from build123d import *

# Parameters (mm, degrees)
SKETCH1_R               = 2.000000064
BOSS_EXTRUDE1_DEPTH     = 3.175
SKETCH2_R               = 2.000000064
BOSS_EXTRUDE2_DEPTH     = 3.175
SKETCH1_2_R             = 2.000000064
CUT_EXTRUDE4_DEPTH      = 3.81
CUT_EXTRUDE4_DEPTH_BACK = 3.81


with BuildPart() as part:
    # Sketch1 → Boss-Extrude1 (new body)
    with BuildSketch(Plane(origin=(0, 0, 0), x_dir=(1, 0, 0), z_dir=(0, 1, 0))):
        with BuildLine():
            Line((-50.8, 6.35), (50.8, 6.35))
            ThreePointArc((50.8, 6.35), (57.15, 0), (50.8, -6.35))
            Line((50.8, -6.35), (-50.8, -6.35))
            ThreePointArc((-50.8, -6.35), (-57.15, 0), (-50.8, 6.35))
        make_face()
        with Locations((-50.8, 0)):
            Circle(SKETCH1_R, mode=Mode.SUBTRACT)
        with Locations((50.8, 0)):
            Circle(SKETCH1_R, mode=Mode.SUBTRACT)
    extrude(amount=BOSS_EXTRUDE1_DEPTH)

    # Sketch2 → Boss-Extrude2 (add)
    with BuildSketch(Plane(origin=(0, 0, 0), x_dir=(1, 0, 0), z_dir=(0, 1, 0))):
        with BuildLine():
            Line((-141.963181024, -45.300738686), (-53.975, 5.499261314))
            ThreePointArc((-53.975, 5.499261314), (-45.300738686, 3.175), (-47.625, -5.499261314))
            Line((-47.625, -5.499261314), (-135.613181024, -56.299261314))
            ThreePointArc((-135.613181024, -56.299261314), (-144.287442339, -53.975), (-141.963181024, -45.300738686))
        make_face()
        with Locations((-138.788181024, -50.8)):
            Circle(SKETCH2_R, mode=Mode.SUBTRACT)
    extrude(amount=BOSS_EXTRUDE2_DEPTH)

    # Sketch1_2 → Cut-Extrude4 (cut, two sides)
    with BuildSketch(Plane(origin=(0, 0, 0), x_dir=(1, 0, 0), z_dir=(0, 1, 0))) as cut_extrude4_sk:
        with Locations((-50.8, 0)):
            Circle(SKETCH1_2_R)
    extrude(amount=CUT_EXTRUDE4_DEPTH, mode=Mode.SUBTRACT)
    extrude(cut_extrude4_sk.sketch, amount=-CUT_EXTRUDE4_DEPTH_BACK, mode=Mode.SUBTRACT)


solid = part.part
Model file for the job. Use its own axes, mm. Give positions to 0.01 mm unless a question says otherwise; leave off trailing zeros. Write each loop counter-clockwise with the first axis right and the second up, starting at its lowest first coordinate (ties: lowest second). Pieces come first, ordered by that corner, then holes. Notation, with made-up numbers: (6, -40) - (64, -40) arc R21 cw to (64, -7) - close; hole circle Ø10 at (43, 32.25). An arc over 180 degrees is marked (long way). Answer as CSV lines item,"result".
1. Band-saw the part on C-C (z = 50.8). Write the cut outline in (x, y) (3 decimals), and give its area (3 significant figures).
Responses:
outline,"(-145.138, 0) - (-140.788, 0) - (-140.788, 3.175) - (-145.138, 3.175) - close; (-136.788, 0) - (-126.088, 0) - (-126.088, 3.175) - (-136.788, 3.175) - close"
area,"47.8 mm2"
2. Band-saw the part on A-A (y = 0.95). Write the cut outline in (x, z) (3 decimals).
Responses:
outline,"(-141.963, 45.301) - (-53.975, -5.499) arc R6.35 ccw to (-50.8, -6.35) - (50.8, -6.35) arc R6.35 ccw to (50.8, 6.35) - (-49.099, 6.35) - (-135.613, 56.299) arc R6.35 ccw to start; hole circle Ø4 at (-138.788, 50.8); hole circle Ø4 at (-50.8, 0); hole circle Ø4 at (50.8, 0)"
3. Band-saw the part on B-B (z = 0). Write the cut outline in (x, y) (3 decimals), and give its area (3 significant figures).
Responses:
outline,"(-63.5, 0) - (-52.8, 0) - (-52.8, 3.175) - (-63.5, 3.175) - close; (-48.8, 0) - (48.8, 0) - (48.8, 3.175) - (-48.8, 3.175) - close; (52.8, 0) - (57.15, 0) - (57.15, 3.175) - (52.8, 3.175) - close"
area,"358 mm2"
4. Two-plate mould, pull along X, no slides. Class faces 1 (the face through (-144.216, 1.565, 54.095)), 2 (the face through (-51, 3.175, 6)), 3 (the face through (48.802, 1.565, -0.088)): +X half, -X half, draft (parallel to the pull), parting line (faces both ways), or undercut.
Responses:
face 1,"parting line"
face 2,"draft"
face 3,"undercut"
5. Band-saw the part on D-D (x = -33.5). Write the cut outline in (y, z) (3 decimals), and give its area (3 significant figures).
Responses:
outline,"(0, -6.35) - (3.175, -6.35) - (3.175, 6.35) - (0, 6.35) - close"
area,"40.3 mm2"
6. Drill centre lines: L1, parallel to X at y = 0.6, z = 0.5; L2, parallel to X at y = 0.9, z = 0; L3, parallel to Z at x = -6.5, y = 1.75. Where is each one in solid material? Low to high. Write a range as [from, to].
Responses:
L1,"x = [-64.37, -52.74], [-48.86, 48.86], [52.74, 57.13]"
L2,"x = [-63.5, -52.8], [-48.8, 48.8], [52.8, 57.15]"
L3,"z = [-6.35, 6.35]"
7. Pin check, flat tip, straight feed: pin 1 (4 mm diameter, centred on x = -103.5, z = 42, fed in from +Y). Stop position of the tip, or through.
Responses:
pin 1,"passes through"
